The model under review builds one solid part; all positions refer to its coordinate system, in mm. A direction names the side the tool comes from. Coordinates: 2 decimals unless noted, no trailing zeros. Write each loop counter-clockwise with the first axis right and the second up, starting at its lowest first coordinate (ties: lowest second). Pieces come first, ordered by that corner, then holes.
1) For line 1 (Y direction, x = -17.5, z = 6); line 2 (Y direction, x = -33, z = 14.5), list the stretches that pass through material, from the lowest coordinate up.
2) Machinability: for faces 1 (the cylindrical face through (-44.796, 32.025, 46.332)), 2 (the flat face through (-33, 29, 95.25)), which of the approach directions +Z, -Z, +X, -X, +Y, -Y give a long, thin tool a straight path to every point of the face, cutting with its end or side? Answer none if there is none.
3) Add section D-D, the plane y = 37.25. State the section outline as (x, z) points.
4) Add section B-B, the plane y = 33. State the section outline as (x, z) points, then the cut area to 3 significant figures.
5) Add section A-A, the plane z = 79. State the section outline as (x, y) points (3 decimals), then the cut area to 3 significant figures.
6) Add section C-C, the plane x = -43. State the section outline as (y, z) points.
7) For P1, Ø3, axis at x = -49, y = 32.5, coming from the -Z side, flat-tipped, find the tip position at first contact; note if it passes through.
8) Mouldability with a two-part tool opening along Y and no side actions: class faces 3 (the flat face through (-16.999, 31.796, 46.958)), 4 (the flat face through (-48, 32, 93.98)), 5 (the flat face through (-18, 25.535, 47)), 6 (the flat face through (-52.413, 32, 47)) as released by +Y, released by -Y, zero draft, split by the parting line, or undercut.
from build123d import *

# Parameters (mm, degrees)
F1_DEPTH = 95.25
F3_DEPTH = 93.98


with BuildPart() as f1:
    # F0 (on Top) → F1 (new body)
    with BuildSketch(Plane.XY):
        Polygon((-52.412679, 38.235107), (-52.412679, 25.535107), (17.437321, 25.535107), align=None)
    extrude(amount=F1_DEPTH)

    # F2 (on face) → F3 (cut)
    with BuildSketch(Plane(origin=(0, 0, 0), x_dir=(1, 0, 0), z_dir=(0, 0, -1))):
        with BuildLine():
            ThreePointArc((-44.792679, -31.885107), (-47.967679, -28.710107), (-51.142679, -31.885107))
            ThreePointArc((-51.142679, -31.885107), (-47.967679, -35.060107), (-44.792679, -31.885107))
        make_face()
    extrude(amount=-F3_DEPTH, mode=Mode.SUBTRACT)


solid = f1.part
Geometry results:
1. line 1: y = 25.54 to 31.89
1. line 2: y = 25.54 to 34.71
2. face 1: -Z
2. face 2: +Z, +X, -X, +Y, -Y
3. outline: (-52.41, 0) - (-46.99, 0) - (-46.99, 95.25) - (-52.41, 95.25) - close
4. outline: (-52.41, 0) - (-50.94, 0) - (-50.94, 93.98) - (-44.99, 93.98) - (-44.99, 0) - (-23.62, 0) - (-23.62, 95.25) - (-52.41, 95.25) - close
4. area: 2,180 mm2
5. outline: (-52.413, 25.535) - (17.437, 25.535) - (-52.413, 38.235) - close; hole circle Ø6.35 at (-47.968, 31.885)
5. area: 412 mm2
6. outline: (25.54, 0) - (36.52, 0) - (36.52, 95.25) - (25.54, 95.25) - close
7. P1: stops at z = 93.98
8. face 3: released by +Y
8. face 4: undercut
8. face 5: released by -Y
8. face 6: zero draft
